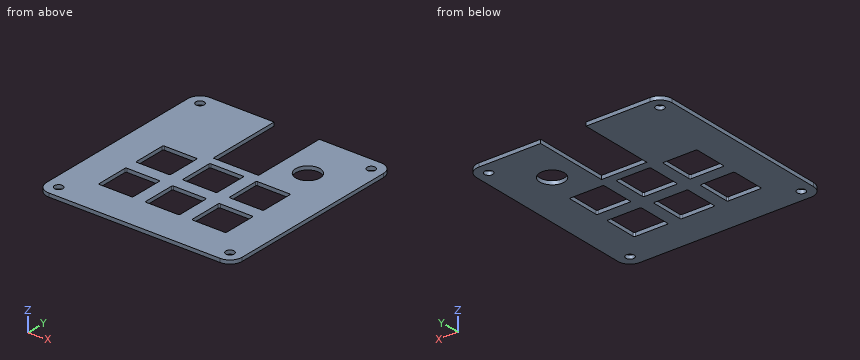
Autodesk Fusion 360 part; units mm, degrees
sketch "Sketch1" plane through (0, 0, 0) normal (0, 0, 1) x (1, 0, 0)
  line L0 (3.025, -2.525) -> (16.025, -2.525)
  line L1 (3.025, -16.525) -> (16.025, -16.525)
  line L2 (2.525, -3.025) -> (2.525, -16.025)
  line L3 (16.525, -3.025) -> (16.525, -16.025)
  arc A0 (3.025, -2.525) -> (2.525, -3.025) centre (3.025, -3.025) ccw
  arc A1 (16.525, -3.025) -> (16.025, -2.525) centre (16.025, -3.025) ccw
  arc A2 (2.525, -16.025) -> (3.025, -16.525) centre (3.025, -16.025) ccw
  arc A3 (16.025, -16.525) -> (16.525, -16.025) centre (16.025, -16.025) ccw
  line L4 (22.075, -2.525) -> (35.075, -2.525)
  line L5 (22.075, -16.525) -> (35.075, -16.525)
  line L6 (21.575, -3.025) -> (21.575, -16.025)
  line L7 (35.575, -3.025) -> (35.575, -16.025)
  arc A4 (22.075, -2.525) -> (21.575, -3.025) centre (22.075, -3.025) ccw
  arc A5 (35.575, -3.025) -> (35.075, -2.525) centre (35.075, -3.025) ccw
  arc A6 (21.575, -16.025) -> (22.075, -16.525) centre (22.075, -16.025) ccw
  arc A7 (35.075, -16.525) -> (35.575, -16.025) centre (35.075, -16.025) ccw
  line L8 (41.125, -2.525) -> (54.125, -2.525)
  line L9 (41.125, -16.525) -> (54.125, -16.525)
  line L10 (40.625, -3.025) -> (40.625, -16.025)
  line L11 (54.625, -3.025) -> (54.625, -16.025)
  arc A8 (41.125, -2.525) -> (40.625, -3.025) centre (41.125, -3.025) ccw
  arc A9 (54.625, -3.025) -> (54.125, -2.525) centre (54.125, -3.025) ccw
  arc A10 (40.625, -16.025) -> (41.125, -16.525) centre (41.125, -16.025) ccw
  arc A11 (54.125, -16.525) -> (54.625, -16.025) centre (54.125, -16.025) ccw
  line L12 (3.025, -21.575) -> (16.025, -21.575)
  line L13 (3.025, -35.575) -> (16.025, -35.575)
  line L14 (2.525, -22.075) -> (2.525, -35.075)
  line L15 (16.525, -22.075) -> (16.525, -35.075)
  arc A12 (3.025, -21.575) -> (2.525, -22.075) centre (3.025, -22.075) ccw
  arc A13 (16.525, -22.075) -> (16.025, -21.575) centre (16.025, -22.075) ccw
  arc A14 (2.525, -35.075) -> (3.025, -35.575) centre (3.025, -35.075) ccw
  arc A15 (16.025, -35.575) -> (16.525, -35.075) centre (16.025, -35.075) ccw
  line L16 (22.075, -21.575) -> (35.075, -21.575)
  line L17 (22.075, -35.575) -> (35.075, -35.575)
  line L18 (21.575, -22.075) -> (21.575, -35.075)
  line L19 (35.575, -22.075) -> (35.575, -35.075)
  arc A16 (22.075, -21.575) -> (21.575, -22.075) centre (22.075, -22.075) ccw
  arc A17 (35.575, -22.075) -> (35.075, -21.575) centre (35.075, -22.075) ccw
  arc A18 (21.575, -35.075) -> (22.075, -35.575) centre (22.075, -35.075) ccw
  arc A19 (35.075, -35.575) -> (35.575, -35.075) centre (35.075, -35.075) ccw
  line L20 (41.125, -21.575) -> (54.125, -21.575)
  line L21 (41.125, -35.575) -> (54.125, -35.575)
  line L22 (40.625, -22.075) -> (40.625, -35.075)
  line L23 (54.625, -22.075) -> (54.625, -35.075)
  arc A20 (41.125, -21.575) -> (40.625, -22.075) centre (41.125, -22.075) ccw
  arc A21 (54.625, -22.075) -> (54.125, -21.575) centre (54.125, -22.075) ccw
  arc A22 (40.625, -35.075) -> (41.125, -35.575) centre (41.125, -35.075) ccw
  arc A23 (54.125, -35.575) -> (54.625, -35.075) centre (54.125, -35.075) ccw
  line L24 (-11.052, 31.916) -> (68.948, 31.916)
  line L25 (68.948, 31.916) -> (68.948, -50.084)
  line L26 (68.948, -50.084) -> (-11.052, -50.084)
  line L27 (-11.052, -50.084) -> (-11.052, 31.916)
  line L28 (20.198, 31.916) -> (38.698, 31.916)
  line L29 (38.698, 31.916) -> (38.698, 0.916)
  line L30 (38.698, 0.916) -> (20.198, 0.916)
  line L31 (20.198, 0.916) -> (20.198, 31.916)
  circle A24 centre (-6.052, 26.916) radius 1.7
  circle A25 centre (-6.052, -45.084) radius 1.7
  circle A26 centre (63.948, -45.084) radius 1.7
  circle A27 centre (63.948, 26.916) radius 1.7
  dimension "d1" = 80
  dimension "d2" = 82
  dimension "d4" = 13.577
  dimension "d5" = 14.509
  dimension "d6" = 18.5
  dimension "d7" = 31
  dimension "d8" = 31.25
  dimension "d9" = 3.4
  dimension "d10" = 5
  dimension "d11" = 5
  dimension "d12" = 3.4
  dimension "d13" = 5
  dimension "d14" = 5
  dimension "d15" = 3.4
  dimension "d16" = 5
  dimension "d17" = 5
  dimension "d18" = 3.4
  dimension "d19" = 5
  dimension "d20" = 5
extrude "Extrude1" add sketch "Sketch1" along normal blind 1.5 contours L24 L25 L26 L27 L29 L30 L31
fillet "Fillet1" radius 5 4 edges at (-11.052, -50.084, 0.75) (-11.052, 31.916, 0.75) (68.948, -50.084, 0.75) (68.948, 31.916, 0.75)
sketch "Sketch2" plane through (0, 0, 1.5) normal (0, 0, 1) x (-1, 0, 0)
  arc A0 (-68.948, -26.916) -> (-63.948, -31.916) centre (-63.948, -26.916) ccw
  line L0 (-63.948, -31.916) -> (-38.698, -31.916)
  line L1 (-38.698, -31.916) -> (-38.698, -0.916)
  line L2 (-38.698, -0.916) -> (-20.198, -0.916)
  line L3 (-20.198, -0.916) -> (-20.198, -31.916)
  line L4 (-20.198, -31.916) -> (6.052, -31.916)
  arc A1 (6.052, -31.916) -> (11.052, -26.916) centre (6.052, -26.916) ccw
  line L5 (11.052, -26.916) -> (11.052, 45.084)
  arc A2 (11.052, 45.084) -> (6.052, 50.084) centre (6.052, 45.084) ccw
  line L6 (6.052, 50.084) -> (-63.948, 50.084)
  arc A3 (-63.948, 50.084) -> (-68.948, 45.084) centre (-63.948, 45.084) ccw
  line L7 (-68.948, 45.084) -> (-68.948, -26.916)
  arc A4 (-41.125, 2.525) -> (-40.625, 3.025) centre (-41.125, 3.025) ccw
  line L8 (-41.125, 2.525) -> (-54.125, 2.525)
  arc A5 (-54.625, 3.025) -> (-54.125, 2.525) centre (-54.125, 3.025) ccw
  line L9 (-54.625, 3.025) -> (-54.625, 16.025)
  arc A6 (-54.125, 16.525) -> (-54.625, 16.025) centre (-54.125, 16.025) ccw
  line L10 (-54.125, 16.525) -> (-41.125, 16.525)
  arc A7 (-40.625, 16.025) -> (-41.125, 16.525) centre (-41.125, 16.025) ccw
  line L11 (-40.625, 16.025) -> (-40.625, 3.025)
  arc A8 (-22.075, 2.525) -> (-21.575, 3.025) centre (-22.075, 3.025) ccw
  line L12 (-22.075, 2.525) -> (-35.075, 2.525)
  arc A9 (-35.575, 3.025) -> (-35.075, 2.525) centre (-35.075, 3.025) ccw
  line L13 (-35.575, 3.025) -> (-35.575, 16.025)
  arc A10 (-35.075, 16.525) -> (-35.575, 16.025) centre (-35.075, 16.025) ccw
  line L14 (-35.075, 16.525) -> (-22.075, 16.525)
  arc A11 (-21.575, 16.025) -> (-22.075, 16.525) centre (-22.075, 16.025) ccw
  line L15 (-21.575, 16.025) -> (-21.575, 3.025)
  circle A12 centre (-63.948, 45.084) radius 1.7
  arc A13 (-3.025, 21.575) -> (-2.525, 22.075) centre (-3.025, 22.075) ccw
  line L16 (-3.025, 21.575) -> (-16.025, 21.575)
  arc A14 (-16.525, 22.075) -> (-16.025, 21.575) centre (-16.025, 22.075) ccw
  line L17 (-16.525, 22.075) -> (-16.525, 35.075)
  arc A15 (-16.025, 35.575) -> (-16.525, 35.075) centre (-16.025, 35.075) ccw
  line L18 (-16.025, 35.575) -> (-3.025, 35.575)
  arc A16 (-2.525, 35.075) -> (-3.025, 35.575) centre (-3.025, 35.075) ccw
  line L19 (-2.525, 35.075) -> (-2.525, 22.075)
  arc A17 (-3.025, 2.525) -> (-2.525, 3.025) centre (-3.025, 3.025) ccw
  line L20 (-3.025, 2.525) -> (-16.025, 2.525)
  arc A18 (-16.525, 3.025) -> (-16.025, 2.525) centre (-16.025, 3.025) ccw
  line L21 (-16.525, 3.025) -> (-16.525, 16.025)
  arc A19 (-16.025, 16.525) -> (-16.525, 16.025) centre (-16.025, 16.025) ccw
  line L22 (-16.025, 16.525) -> (-3.025, 16.525)
  arc A20 (-2.525, 16.025) -> (-3.025, 16.525) centre (-3.025, 16.025) ccw
  line L23 (-2.525, 16.025) -> (-2.525, 3.025)
  circle A21 centre (6.052, 45.084) radius 1.7
  arc A22 (-41.125, 21.575) -> (-40.625, 22.075) centre (-41.125, 22.075) ccw
  line L24 (-41.125, 21.575) -> (-54.125, 21.575)
  arc A23 (-54.625, 22.075) -> (-54.125, 21.575) centre (-54.125, 22.075) ccw
  line L25 (-54.625, 22.075) -> (-54.625, 35.075)
  arc A24 (-54.125, 35.575) -> (-54.625, 35.075) centre (-54.125, 35.075) ccw
  line L26 (-54.125, 35.575) -> (-41.125, 35.575)
  arc A25 (-40.625, 35.075) -> (-41.125, 35.575) centre (-41.125, 35.075) ccw
  line L27 (-40.625, 35.075) -> (-40.625, 22.075)
  circle A26 centre (6.052, -26.916) radius 1.7
  arc A27 (-22.075, 21.575) -> (-21.575, 22.075) centre (-22.075, 22.075) ccw
  line L28 (-22.075, 21.575) -> (-35.075, 21.575)
  arc A28 (-35.575, 22.075) -> (-35.075, 21.575) centre (-35.075, 22.075) ccw
  line L29 (-35.575, 22.075) -> (-35.575, 35.075)
  arc A29 (-35.075, 35.575) -> (-35.575, 35.075) centre (-35.075, 35.075) ccw
  line L30 (-35.075, 35.575) -> (-22.075, 35.575)
  arc A30 (-21.575, 35.075) -> (-22.075, 35.575) centre (-22.075, 35.075) ccw
  line L31 (-21.575, 35.075) -> (-21.575, 22.075)
  circle A31 centre (-63.948, -26.916) radius 1.7
  circle A32 centre (-50.098, -11.875) radius 5
  dimension "d28" = 10
  dimension "d29" = 14.4
  dimension "d30" = 11.4
extrude "Extrude2" cut sketch "Sketch2" against normal blind 5 contours A32
Part model, mm, in its own coordinate system. Coordinates: 2 decimals unless noted, no trailing zeros. Order: outer loops, then holes, each group sorted by start corner. A loop starts at its lowest first (then second) coordinate and runs counter-clockwise, first axis right, second up.
(1) Probe L1, parallel to Y at x = 13, z = 1.2 (3 decimals); L2, parallel to X at y = -34, z = 1.3 (3 decimals); L3, parallel to Y at x = 27.5, z = 1.2 (3 decimals). List the from-to ranges inside material, lowest first.
Check sheet entries:
L1: y = -50.084 to -35.575, -21.575 to -16.525, -2.525 to 31.916
L2: x = -11.052 to 2.525, 16.525 to 21.575, 35.575 to 40.625, 54.625 to 68.948
L3: y = -50.084 to -35.575, -21.575 to -16.525, -2.525 to 0.916
(2) Pin check, flat tips, straight feed: pin 1 Ø3 at (x, y) = (63.948, -45.084) entering from -Z; pin 2 Ø0.8 at (x, z) = (30, 0.5) entering from +Y. Stop position of each tip, or through.
Check sheet entries:
pin 1: passes through
pin 2: stops at y = 0.92
(3) Slice it at A-A, the plane y = -10.5. Write the cut outline in (x, z) (3 decimals), and give its area (3 significant figures).
Check sheet entries:
outline: (-11.052, 0) - (2.525, 0) - (2.525, 1.5) - (-11.052, 1.5) - close; (16.525, 0) - (21.575, 0) - (21.575, 1.5) - (16.525, 1.5) - close; (35.575, 0) - (40.625, 0) - (40.625, 1.5) - (35.575, 1.5) - close; (54.625, 0) - (68.948, 0) - (68.948, 1.5) - (54.625, 1.5) - close
area: 57.0 mm2
(4) Slice it at D-D, the plane x = 53. Write the cut outline in (y, z) (3 decimals), and give its area (3 significant figures).
Check sheet entries:
outline: (-50.084, 0) - (-35.575, 0) - (-35.575, 1.5) - (-50.084, 1.5) - close; (-21.575, 0) - (-16.525, 0) - (-16.525, 1.5) - (-21.575, 1.5) - close; (-2.525, 0) - (7.803, 0) - (7.803, 1.5) - (-2.525, 1.5) - close; (15.947, 0) - (31.916, 0) - (31.916, 1.5) - (15.947, 1.5) - close
area: 68.8 mm2
(5) Slice it at C-C, the plane y = 24. Write the cut outline in (x, z).
Check sheet entries:
outline: (-11.05, 0) - (20.2, 0) - (20.2, 1.5) - (-11.05, 1.5) - close; (38.7, 0) - (68.95, 0) - (68.95, 1.5) - (38.7, 1.5) - close
(6) Slice it at B-B, the plane x = 9.5. Write the cut outline in (y, z) (3 decimals).
Check sheet entries:
outline: (-50.084, 0) - (-35.575, 0) - (-35.575, 1.5) - (-50.084, 1.5) - close; (-21.575, 0) - (-16.525, 0) - (-16.525, 1.5) - (-21.575, 1.5) - close; (-2.525, 0) - (31.916, 0) - (31.916, 1.5) - (-2.525, 1.5) - close
